Verification items for the finished model (mm, model axes). Face numbers are marked on the shaded views. A direction names the side the tool comes from. Give positions to 0.01 mm unless a question says otherwise; leave off trailing zeros. One line per question, with ' | ' between items. Start each with the question number.
Q1. Material ranges on probe 1 along Y at (x, z) = (0, 10); probe 2 along Y at (x, z) = (10, 75); probe 3 along Z at (x, y) = (-13, 22), recorded low to high. Write a range as [from, to].
Q2. Go/stop test with flat-tipped pins: pin 1 (6 mm diameter, centred on x = -18.5, y = 28, fed in from -Z); pin 2 (3 mm diameter, centred on x = -9, z = 88.5, fed in from +Y); pin 3 (6 mm diameter, centred on x = -10.5, y = 29.5, fed in from +Z). Record where each tip stops, or that it passes through.
Q3. Mould release check, pull along Y, two halves, no side actions. Record for the marked faces 3 and 4: released by +Y, released by -Y, zero draft, split by the parting line, or undercut.
Q4. Access from +Z, -Z, +X, -X, +Y, -Y to the whole of each face (thin tool, end or side, straight path). Record for the marked faces 1 and 2.
from build123d import *

# Parameters (mm, degrees)
ESQUISSE6_R        = 25
ESQUISSE6_R_2      = 24
ESQUISSE8_R        = 26
ESQUISSE8_R_2      = 24
EXTRU_MINCE1_DEPTH = 1
EXTRU_MINCE2_START = 30
ESQUISSE9_R        = 26
ESQUISSE9_R_2      = 25
EXTRU_MINCE2_DEPTH = 30
CONG_1_R           = 1
CONG_2_R           = 1


with BuildPart() as part:
    # Balayage-Mince2: sweep along a path in Esquisse7
    with BuildLine(Plane(origin=(0, 0, 0), x_dir=(0, 0, -1), z_dir=(1, 0, 0))) as balayage_mince2_path:
        Line((0, 0), (-42.573593129, 0))
        ThreePointArc((-42.573593129, 0), (-54.0540961, 2.283614025), (-63.786796564, 8.786796564))
        Line((-63.786796564, 8.786796564), (-71.970562748, 16.970562748))
    # Esquisse6 → Balayage-Mince2 (sweep)
    with BuildSketch(Plane.XY):
        Circle(ESQUISSE6_R)
        Circle(ESQUISSE6_R_2, mode=Mode.SUBTRACT)
    sweep(path=balayage_mince2_path.line)



with BuildPart() as body_2:
    # Esquisse8 → Extru.-Mince1 (new body)
    with BuildSketch(Plane(origin=(0, 44.470562748, 44.470562748), x_dir=(1, 0, 0), z_dir=(0, 0.7071067811865487, 0.7071067811865464))):
        with Locations((0, -38.890872965)):
            Circle(ESQUISSE8_R)
        with Locations((0, -38.890872965)):
            Circle(ESQUISSE8_R_2, mode=Mode.SUBTRACT)
    extrude(amount=EXTRU_MINCE1_DEPTH)


with BuildPart() as part_1:
    add(part.part)

    add(body_2.part)  # Extru.-Mince2 merges body 2
    # Esquisse9 → Extru.-Mince2 (add)
    with BuildSketch(Plane(origin=(0, 45.17766953, 45.17766953), x_dir=(1, 0, 0), z_dir=(0, 0.7071067811865487, 0.7071067811865464)).offset(EXTRU_MINCE2_START)):
        with Locations((0, -38.890872965)):
            Circle(ESQUISSE9_R)
        with Locations((0, -38.890872965)):
            Circle(ESQUISSE9_R_2, mode=Mode.SUBTRACT)
    extrude(amount=-EXTRU_MINCE2_DEPTH)

    # Congé1
    cong_1_edges = [part_1.edges().sort_by_distance(p)[0] for p in [
        (-25, 16.970562748, 71.970562748),
    ]]
    fillet(cong_1_edges, radius=CONG_1_R - 0.0001)  # a hair under: the kernel refuses the full size

    # Congé2
    cong_2_edges = [part_1.edges().sort_by_distance(p)[0] for p in [
        (-26, 16.970562748, 71.970562748),
    ]]
    fillet(cong_2_edges, radius=CONG_2_R)


solid = part_1.part
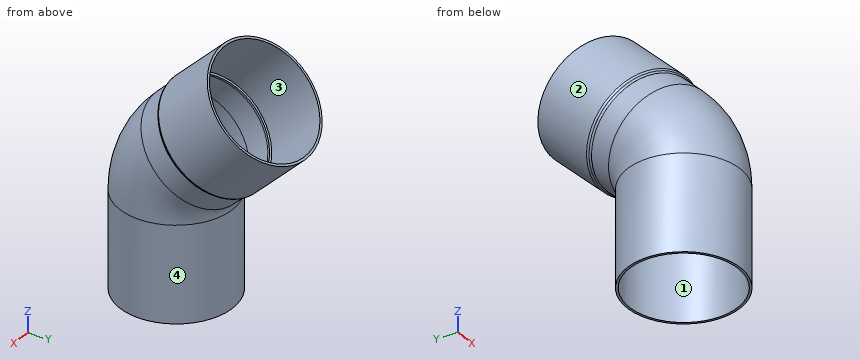
Filled in:
1) probe 1: [-25, -24], [24, 25] | probe 2: [-11.81, -10.42], [52.4, 53.94] | probe 3: [45.85, 48.28], [107.2, 108.84]
2) pin 1: z = 54.15 | pin 2: y = 2.38 | pin 3: z = 57.76
3) face 3: undercut | face 4: split by the parting line
4) face 1: -Z | face 2: none
